Can you work these out from the model? Positions are in its coordinate system, mm. A direction names the side the tool comes from. Coordinates: 2 decimals unless noted, no trailing zeros. Order: outer loops, then holes, each group sorted by start corner. A loop starts at its lowest first (then second) coordinate and runs counter-clockwise, first axis right, second up. Notation, with made-up numbers: (88.25, 47.5) -> (144.25, 47.5) arc R22 ccw to (144.25, 61.5) -> close; hole circle Ø2 at (-22, -0.75). An arc over 180 degrees is marked (long way). Answer as a JSON object with one key per item and string values. Group by question number.
(1) I want a section at A-A, the plane y = 5. List the corners of the cut face in (x, z) for me, plus the area to 3 significant figures.
(2) I want a section at D-D, the plane y = 68. List the corners of the cut face in (x, z) for me, plus the area to 4 significant figures.
(3) I want a section at C-C, the plane z = -220. List the corners of the cut face in (x, y) for me.
(4) For pin 1 (12 mm diameter, centred on y = -32.5, z = 15.5, fed in from -X); pin 2 (12 mm diameter, centred on y = -72.5, z = -171.5, fed in from -X); pin 3 (5 mm diameter, centred on y = 50, z = -86.5, fed in from -X), each with a flat end and sliding along its axis, tell me the tip position at first contact or that it passes through.
(5) I need wall thicknesses on line 1 (Z direction, x = -104.5, y = 14); line 2 (Z direction, x = -25.5, y = -47); line 3 (Y direction, x = 95, z = -417). Which ranges of each line are inside material? Lowest first, please.
(6) I want a section at B-B, the plane x = 74.5. List the corners of the cut face in (y, z) for me, plus the area to 3 significant figures.
(7) Which directions (+Z, -Z, +X, -X, +Y, -Y) give clear straight access to the entire face, cutting with the end or side of a thin tool? Please do faces 1 (the flat face through (2, 0, -350.464)), 2 (the flat face through (2, 14.333, -386)), 3 (the flat face through (-150, -2, 20)), 4 (the flat face through (2, 0, -420.728)).
(8) If we mould it in two halves opening along X, with no side actions, what happens to faces 5 (the flat face through (-127.815, -2.1, -238.29)), 6 (the flat face through (2, -14.333, -386)), 7 (the flat face through (174, 2, -470)), 8 (the flat face through (150, -2, 20))? For each: pulls with the +X half, pulls with the -X half, needs draft (parallel to the pull), parting line crosses it, or undercut.
from build123d import *

# Parameters (mm, degrees)
F0_W          = 300
F0_H          = 300
F1_DEPTH      = 40
F4_W          = 45
F4_H          = 300
F3_W          = 50
F3_H          = 300
F7_W          = 28.6667700857
F7_H          = 70.264339447
F8_DEPTH      = 150
F8_DEPTH_BACK = 150


# Not quite as in the source:
# - an extrude ends at something that could not be found from the text; its depth is read off the source's solid


with BuildPart() as f1:
    # F0 (on Top) → F1 (new body)
    with BuildSketch(Plane.XY):
        Rectangle(F0_W, F0_H)
    extrude(amount=F1_DEPTH)

    # F4 (on face) → F5 section 0
    with BuildSketch(Plane(origin=(0, 0, 0), x_dir=(1, 0, 0), z_dir=(0, 0, -1))):
        with Locations((127.5, 0)):
            Rectangle(F4_W, F4_H)
    # F3 (on offset) → F5 section 1
    with BuildSketch(Plane(origin=(0, 0, -470), x_dir=(1, 0, 0), z_dir=(0, 0, -1))):
        with Locations((175, 0)):
            Rectangle(F3_W, F3_H)
    loft()

    # F6: F1 across plane


with BuildPart() as f1_1:
    add(f1.part)
    add(f1.part.mirror(Plane.YZ))

    # F7 (on Right) → F8 (join, two sides)
    with BuildSketch(Plane.YZ) as f8_sk:
        with Locations((0, -385.5957090855)):
            Rectangle(F7_W, F7_H)
    extrude(amount=F8_DEPTH)
    extrude(f8_sk.sketch, amount=-F8_DEPTH_BACK)


solid = f1_1.part
Computed values:
{
 "1": {"outline": "(-200, -470) -> (-150, -470) -> (-145.28, -420.73) -> (145.28, -420.73) -> (150, -470) -> (200, -470) -> (150, 0) -> (150, 40) -> (-150, 40) -> (-150, 0) -> close; hole (-138.56, -350.46) -> (138.56, -350.46) -> (105, 0) -> (-105, 0) -> close", "area": "76,600 mm2"},
 "2": {"outline": "(-200, -470) -> (-150, -470) -> (-105, 0) -> (105, 0) -> (150, -470) -> (200, -470) -> (150, 0) -> (150, 40) -> (-150, 40) -> (-150, 0) -> close", "area": "56,650 mm2"},
 "3": {"outline": "(-173.4, -150) -> (-126.06, -150) -> (-126.06, 150) -> (-173.4, 150) -> close; (126.06, -150) -> (173.4, -150) -> (173.4, 150) -> (126.06, 150) -> close"},
 "4": {"pin 1": "stops at x = -150", "pin 2": "stops at x = -168.88", "pin 3": "stops at x = -159.47"},
 "5": {"line 1": "z = -420.73 to -350.46, 0 to 40", "line 2": "z = 0 to 40", "line 3": "y = -14.33 to 14.33"},
 "6": {"outline": "(-150, 0) -> (150, 0) -> (150, 40) -> (-150, 40) -> close; (-14.33, -420.73) -> (14.33, -420.73) -> (14.33, -350.46) -> (-14.33, -350.46) -> close", "area": "14,000 mm2"},
 "7": {"face 1": "+Y, -Y", "face 2": "-Z, +Y", "face 3": "+Z, -X, +Y, -Y", "face 4": "-Z, +Y, -Y"},
 "8": {"face 5": "undercut", "face 6": "undercut", "face 7": "needs draft", "face 8": "pulls with the +X half"}
}
